from build123d import *

# Parameters (mm, degrees)
BOSS_EXTRUDE1_DEPTH = 19
SKETCH2_R           = 3
CUT_EXTRUDE1_DEPTH  = 32.4
FILLET1_R           = 5


with BuildPart() as part:
    # Sketch1 → Boss-Extrude1 (new body, symmetric)
    with BuildSketch(Plane.XY):
        Polygon((-15.7, 39.6), (-12.7, 39.6), (-12.7, 4), (12.7, 4), (12.7, 39.6), (15.7, 39.6), (15.7, 0), (-15.7, 0), align=None)
    extrude(amount=BOSS_EXTRUDE1_DEPTH, both=True)

    # Sketch2 → Cut-Extrude1 (cut, through all)
    with BuildSketch(Plane(origin=(15.7, 0, 0), x_dir=(0, 0, -1), z_dir=(1, 0, 0))):
        with Locations((0, 16.7)):
            Circle(SKETCH2_R)
    extrude(amount=-CUT_EXTRUDE1_DEPTH, mode=Mode.SUBTRACT)

    # Fillet1
    fillet1_edges = [part.edges().sort_by_distance(p)[0] for p in [
        (14.2, 39.6, -19),
        (15.7, 0, 0),
        (-15.7, 0, 0),
        (14.2, 39.6, 19),
        (-14.2, 39.6, 19),
        (-14.2, 39.6, -19),
    ]]
    fillet(fillet1_edges, radius=FILLET1_R)


solid = part.part
Work out the finished part from the listing and answer in its coordinate system (mm). A direction names the side the tool comes from. Give positions to 0.01 mm unless a question says otherwise; leave off trailing zeros. Order: outer loops, then holes, each group sorted by start corner. A loop starts at its lowest first (then second) coordinate and runs counter-clockwise, first axis right, second up. Notation, with made-up numbers: (84, 20.25) -> (93, 20.25) arc R21 cw to (93, 39.25) -> close; hole circle Ø11 at (50, 4). An arc over 180 degrees is marked (long way). Answer as a JSON object with one key per item and string values. Group by question number.
1. A flat-ended cylindrical pin translates along its axis: pin 1 Ø1 at (x, z) = (-6.5, -12) entering from +Y. Find the tip coordinate at first contact, or state that the pin passes through.
2. Section B-B on y = 16.7 is taken. Determine the outline of the cut face in (x, z).
3. Consider line 1 along X through (y, z) = (22.5, 16); line 2 along Y through (x, z) = (-5.5, -4); line 3 along Y through (x, z) = (14, 0). Determine where each line is inside the solid, lowest interval first. Write a range as [from, to].
4. Section C-C on y = 21.5 is taken. Determine the outline of the cut face in (x, z), plus the area to 3 significant figures.
5. A tool of negligible diameter and unlimited length cuts with its end or side. For faces 1 (the flat face through (12.7, 22, 0)), 2 (the cylindrical face through (14.22, 38.1, -17.57)), from which of +Z, -Z, +X, -X, +Y, -Y can it reach the whole face along a straight path? Write none if from no direction.
6. The mould has two halves that part along Y. Classify faces 3 (the cylindrical face through (14.22, 38.1, 17.57)), 4 (the flat face through (0, 0, 0)), 5 (the cylindrical face through (-14.179, 19.674, 0.391)): released by +Y, released by -Y, zero draft, split by the parting line, or undercut.
7. Section A-A on z = 0 is taken. Determine the outline of the cut face in (x, y).
8. Section D-D on z = 10 is taken. Determine the outline of the cut face in (x, y), plus the area to 3 significant figures.
Result sheet:
{
 "1": {"pin 1": "stops at y = 4"},
 "2": {"outline": "(-15.7, -19) -> (-12.7, -19) -> (-12.7, -3) -> (-15.7, -3) -> close; (-15.7, 3) -> (-12.7, 3) -> (-12.7, 19) -> (-15.7, 19) -> close; (12.7, -19) -> (15.7, -19) -> (15.7, -3) -> (12.7, -3) -> close; (12.7, 3) -> (15.7, 3) -> (15.7, 19) -> (12.7, 19) -> close"},
 "3": {"line 1": "x = [-15.7, -12.7], [12.7, 15.7]", "line 2": "y = [0, 4]", "line 3": "y = [1.24, 13.7], [19.7, 39.6]"},
 "4": {"outline": "(-15.7, -19) -> (-12.7, -19) -> (-12.7, 19) -> (-15.7, 19) -> close; (12.7, -19) -> (15.7, -19) -> (15.7, 19) -> (12.7, 19) -> close", "area": "228 mm^2"},
 "5": {"face 1": "+Z, -Z, +Y", "face 2": "-Z, +X, -X, +Y"},
 "6": {"face 3": "released by +Y", "face 4": "released by -Y", "face 5": "undercut"},
 "7": {"outline": "(-15.7, 5) arc R5 ccw to (-10.7, 0) -> (10.7, 0) arc R5 ccw to (15.7, 5) -> (15.7, 13.7) -> (12.7, 13.7) -> (12.7, 4) -> (-12.7, 4) -> (-12.7, 13.7) -> (-15.7, 13.7) -> close; (-15.7, 19.7) -> (-12.7, 19.7) -> (-12.7, 39.6) -> (-15.7, 39.6) -> close; (12.7, 19.7) -> (15.7, 19.7) -> (15.7, 39.6) -> (12.7, 39.6) -> close"},
 "8": {"outline": "(-15.7, 5) arc R5 ccw to (-10.7, 0) -> (10.7, 0) arc R5 ccw to (15.7, 5) -> (15.7, 39.6) -> (12.7, 39.6) -> (12.7, 4) -> (-12.7, 4) -> (-12.7, 39.6) -> (-15.7, 39.6) -> close", "area": "328 mm^2"}
}
